from build123d import *

# Parameters (mm, degrees)
SKETCH1_W           = 46
SKETCH1_H           = 25
BOSS_EXTRUDE1_DEPTH = 37
SKETCH2_R           = 10
BOSS_EXTRUDE2_DEPTH = 160
SKETCH3_W           = 37.5
SKETCH3_H           = 36.8
CUT_EXTRUDE1_DEPTH  = 30


with BuildPart() as part:
    # Sketch1 → Boss-Extrude1 (new body)
    with BuildSketch(Plane.XY):
        Rectangle(SKETCH1_W, SKETCH1_H)
    extrude(amount=-BOSS_EXTRUDE1_DEPTH)

    # Sketch2 → Boss-Extrude2 (add)
    with BuildSketch(Plane(origin=(0, 0, -37), x_dir=(-1, 0, 0), z_dir=(0, 0, -1))):
        Circle(SKETCH2_R)
    extrude(amount=BOSS_EXTRUDE2_DEPTH)

    # Sketch3 → Cut-Extrude1 (cut)
    with BuildSketch(Plane.XY):
        with Locations((-0.5, 0)):
            Rectangle(SKETCH3_W, SKETCH3_H)
    extrude(amount=-CUT_EXTRUDE1_DEPTH, mode=Mode.SUBTRACT)


solid = part.part
For this review, take the finished solid that the model builds, in its own axes (mm). A direction names the side the tool comes from. Round coordinates to 2 decimals unless told otherwise and drop trailing zeros. Order: outer loops, then holes, each group sorted by start corner. A loop starts at its lowest first (then second) coordinate and runs counter-clockwise, first axis right, second up. Notation, with made-up numbers: (59, 1.25) -> (92, 1.25) arc R9 cw to (92, 10.25) -> close; hole circle Ø6 at (42, -4). An arc over 180 degrees is marked (long way). Write item = value, one per line. Start each with the question number.
1) To check wall thickness, follow line 1 (Z direction, x = 16.5, y = -5.5); line 2 (Y direction, x = -0.5, z = -175.5); line 3 (Z direction, x = -9, y = -3.5). State the ranges of each line that lie inside material, in increasing order. Write a range as from..to.
2) Insertion check: pin 1 (1 mm diameter, centred on y = 0.5, z = -161, fed in from -X); pin 2 (1 mm diameter, centred on x = 2, z = -157, fed in from +Y); pin 3 (7.5 mm diameter, centred on x = -5.5, y = 4.5, fed in from +Z); pin 4 (8 mm diameter, centred on x = -11, z = -23.5, fed in from +Y). Each pin has a flat end and moves straight along its axis. Give the tip position at first contact, or say it passes through.
3) Take a section at A-A on x = 8. State the section outline as (y, z) points.
4) Take a section at B-B on y = 0. State the section outline as (x, z) points.
5) The part is to be moulded in two halves that separate along X. For faces 1 (the face through (-19.25, 0, -15)), 2 (the face through (23, 0, -18)), 3 (the face through (0, 12.5, -31)), say which applies: +X half, -X half, draft (parallel to the pull), parting line (faces both ways), or undercut.
6) Take a section at C-C on z = -72.5. State the section outline as (x, y) points.
7) Tool access review of faces 4 (the face through (0, 0, -197)), 5 (the face through (18.25, 0, -15)), 6 (the face through (2.17, -9.76, -115.88)): name each direction out of +Z, -Z, +X, -X, +Y, -Y from which nothing blocks a thin tool from reaching the whole face with its end or side.
8) Take a section at D-D on x = 0. State the section outline as (y, z) points, plus the area to 4 significant figures.
Verdict:
q1.line_1 = -37..-30
q1.line_2 = -9.99..9.99
q1.line_3 = -197..-30
q2.pin_1 = -10
q2.pin_2 = 9.89
q2.pin_3 = -30
q2.pin_4 = through
q3.outline = (-12.5, -37) -> (-6, -37) -> (-6, -197) -> (6, -197) -> (6, -37) -> (12.5, -37) -> (12.5, -30) -> (-12.5, -30) -> close
q4.outline = (-23, -37) -> (-10, -37) -> (-10, -197) -> (10, -197) -> (10, -37) -> (23, -37) -> (23, 0) -> (18.25, 0) -> (18.25, -30) -> (-19.25, -30) -> (-19.25, 0) -> (-23, 0) -> close
q5.face_1 = undercut
q5.face_2 = +X half
q5.face_3 = draft
q6.outline = circle Ø20 at (0, 0)
q7.face_4 = -Z, +X, -X, +Y, -Y
q7.face_5 = +Z, +Y, -Y
q7.face_6 = -Z
q8.outline = (-12.5, -37) -> (-10, -37) -> (-10, -197) -> (10, -197) -> (10, -37) -> (12.5, -37) -> (12.5, -30) -> (-12.5, -30) -> close
q8.area = 3,375 mm2
